```python
from build123d import *

# Parameters (mm, degrees)
SKETCH_1_W          = 450
SKETCH_1_H          = 400
EXTRUDE_1_DEPTH     = 6
SKETCH_3_R          = 3.75
SKETCH_3_R_2        = 4.25
CUT_EXTRUDE_2_DEPTH = 50
CUT_EXTRUDE_3_DEPTH = 50
SKETCH_5_W          = 45
SKETCH_5_H          = 45
CUT_EXTRUDE_4_DEPTH = 56
FILLET_1_R          = 5
SKETCH_6_R          = 4.25
CUT_EXTRUDE_5_DEPTH = 90


with BuildPart() as part:
    # 草图1 → 凸台-拉伸1 (new body)
    with BuildSketch(Plane.XY):
        Rectangle(SKETCH_1_W, SKETCH_1_H)
    extrude(amount=EXTRUDE_1_DEPTH)

    # 草图3 → 切除-拉伸2 (cut)
    with BuildSketch(Plane.XY.offset(6)):
        with Locations((205, -180)):
            Circle(SKETCH_3_R)
        with Locations((205, -120)):
            Circle(SKETCH_3_R_2)
        with Locations((145, -180)):
            Circle(SKETCH_3_R_2)
        with Locations((145, 180)):
            Circle(SKETCH_3_R_2)
        with Locations((205, 120)):
            Circle(SKETCH_3_R_2)
        with Locations((205, 180)):
            Circle(SKETCH_3_R)
        with Locations((-205, 180)):
            Circle(SKETCH_3_R)
        with Locations((-205, 120)):
            Circle(SKETCH_3_R_2)
        with Locations((-145, 180)):
            Circle(SKETCH_3_R_2)
        with Locations((-145, -180)):
            Circle(SKETCH_3_R_2)
        with Locations((-205, -120)):
            Circle(SKETCH_3_R_2)
        with Locations((-205, -180)):
            Circle(SKETCH_3_R)
    extrude(amount=-CUT_EXTRUDE_2_DEPTH, mode=Mode.SUBTRACT)

    # 草图4 → 切除-拉伸3 (cut)
    with BuildSketch(Plane.XY.offset(6)):
        with BuildLine():
            Line((100, -12.5), (-100, -12.5))
            ThreePointArc((-100, -12.5), (-112.5, 0), (-100, 12.5))
            Line((-100, 12.5), (100, 12.5))
            ThreePointArc((100, 12.5), (112.5, 0), (100, -12.5))
        make_face()
        with BuildLine():
            Line((100, 47.5), (-100, 47.5))
            ThreePointArc((-100, 47.5), (-112.5, 60), (-100, 72.5))
            Line((-100, 72.5), (100, 72.5))
            ThreePointArc((100, 72.5), (112.5, 60), (100, 47.5))
        make_face()
        with BuildLine():
            Line((100, -47.5), (-100, -47.5))
            ThreePointArc((-100, -47.5), (-112.5, -60), (-100, -72.5))
            Line((-100, -72.5), (100, -72.5))
            ThreePointArc((100, -72.5), (112.5, -60), (100, -47.5))
        make_face()
        with BuildLine():
            Line((100, 127.5), (-100, 127.5))
            ThreePointArc((-100, 127.5), (-112.5, 140), (-100, 152.5))
            Line((-100, 152.5), (100, 152.5))
            ThreePointArc((100, 152.5), (112.5, 140), (100, 127.5))
        make_face()
        with BuildLine():
            Line((100, -127.5), (-100, -127.5))
            ThreePointArc((-100, -127.5), (-112.5, -140), (-100, -152.5))
            Line((-100, -152.5), (100, -152.5))
            ThreePointArc((100, -152.5), (112.5, -140), (100, -127.5))
        make_face()
    extrude(amount=-CUT_EXTRUDE_3_DEPTH, mode=Mode.SUBTRACT)

    # 草图5 → 切除-拉伸4 (cut)
    with BuildSketch(Plane.XY.offset(6)):
        with Locations((202.5, -177.5)):
            Rectangle(SKETCH_5_W, SKETCH_5_H)
        with Locations((-202.5, -177.5)):
            Rectangle(SKETCH_5_W, SKETCH_5_H)
        with Locations((-202.5, 177.5)):
            Rectangle(SKETCH_5_W, SKETCH_5_H)
        with Locations((202.5, 177.5)):
            Rectangle(SKETCH_5_W, SKETCH_5_H)
    extrude(amount=-CUT_EXTRUDE_4_DEPTH, mode=Mode.SUBTRACT)

    # 圆角1
    fillet_1_edges = [part.edges().sort_by_distance(p)[0] for p in [
        (180, 200, 3),
        (225, 155, 3),
        (180, 155, 3),
        (-225, 155, 3),
        (-180, 200, 3),
        (-180, 155, 3),
        (-180, -200, 3),
        (-225, -155, 3),
        (-180, -155, 3),
        (225, -155, 3),
        (180, -200, 3),
        (180, -155, 3),
    ]]
    fillet(fillet_1_edges, radius=FILLET_1_R)

    # 草图6 → 切除-拉伸5 (cut)
    with BuildSketch(Plane(origin=(0, 0, 0), x_dir=(-1, 0, 0), z_dir=(0, 0, -1))):
        with Locations((15, -180)):
            Circle(SKETCH_6_R)
        with Locations((45, -180)):
            Circle(SKETCH_6_R)
        with Locations((75, -180)):
            Circle(SKETCH_6_R)
        with Locations((105, -180)):
            Circle(SKETCH_6_R)
        with Locations((-105, -180)):
            Circle(SKETCH_6_R)
        with Locations((-75, -180)):
            Circle(SKETCH_6_R)
        with Locations((-45, -180)):
            Circle(SKETCH_6_R)
        with Locations((-15, -180)):
            Circle(SKETCH_6_R)
        with Locations((-15, 180)):
            Circle(SKETCH_6_R)
        with Locations((-45, 180)):
            Circle(SKETCH_6_R)
        with Locations((-75, 180)):
            Circle(SKETCH_6_R)
        with Locations((-105, 180)):
            Circle(SKETCH_6_R)
        with Locations((105, 180)):
            Circle(SKETCH_6_R)
        with Locations((75, 180)):
            Circle(SKETCH_6_R)
        with Locations((45, 180)):
            Circle(SKETCH_6_R)
        with Locations((15, 180)):
            Circle(SKETCH_6_R)
        with Locations((-205, -12.5)):
            Circle(SKETCH_6_R)
        with Locations((-205, -37.5)):
            Circle(SKETCH_6_R)
        with Locations((-205, -62.5)):
            Circle(SKETCH_6_R)
        with Locations((-205, -87.5)):
            Circle(SKETCH_6_R)
        with Locations((-205, 87.5)):
            Circle(SKETCH_6_R)
        with Locations((-205, 62.5)):
            Circle(SKETCH_6_R)
        with Locations((-205, 37.5)):
            Circle(SKETCH_6_R)
        with Locations((-205, 12.5)):
            Circle(SKETCH_6_R)
        with Locations((205, 12.5)):
            Circle(SKETCH_6_R)
        with Locations((205, 37.5)):
            Circle(SKETCH_6_R)
        with Locations((205, 62.5)):
            Circle(SKETCH_6_R)
        with Locations((205, 87.5)):
            Circle(SKETCH_6_R)
        with Locations((205, -87.5)):
            Circle(SKETCH_6_R)
        with Locations((205, -62.5)):
            Circle(SKETCH_6_R)
        with Locations((205, -37.5)):
            Circle(SKETCH_6_R)
        with Locations((205, -12.5)):
            Circle(SKETCH_6_R)
    extrude(amount=-CUT_EXTRUDE_5_DEPTH, mode=Mode.SUBTRACT)


solid = part.part
```
Here's how the part is built. I have some questions about the finished solid (model axes, mm). A direction names the side the tool comes from. Coordinates: 2 decimals unless noted, no trailing zeros. Loops run counter-clockwise (first coordinate to the right, second up) from the corner with the lowest first, then second, coordinate; pieces in that order, holes last. Notation, with made-up numbers: (88.5, 35) - (127.5, 35) arc R21 cw to (127.5, 66) - close; hole circle Ø11 at (10, 64.25). An arc over 180 degrees is marked (long way). Return JSON: item names as keys, results as strings. Group by question number.
Item 1: If we section it at B-B on x = -193.5: Write out the boundary of the cut face in (y, z), and give its area (3 significant figures).
Item 2: On a 3-axis mill with a long thin cutter (end or side, diameter ignored), from which of +Z, -Z, +X, -X, +Y, -Y can I reach the whole of each face in a straight line? I mean faces 3 (the face through (-112.497, -0.275, 3.042)), 4 (the face through (-3, -42, 6)). Say none if no direction works.
Item 3: I need wall thicknesses on line 1 (Y direction, x = 84.5, z = 1.8); line 2 (X direction, y = 88, z = 1.1); line 3 (Y direction, x = 145, z = 1.35). Which ranges of each line are inside material? Lowest first, please. Write a range as from..to.
Item 4: We'd pull the mould along Y, two halves only. Please class faces 1 (the face through (-3, -42, 0)), 2 (the face through (112.497, 0.275, 3.042)): +Y half, -Y half, draft (parallel to the pull), parting line (faces both ways), or undercut.
Item 5: Will these pins go through, and if not, where does the flat tip stop? P1, Ø3, axis at y = 183, z = 4.5, coming from the +X side; P2, Ø4, axis at x = 73.5, y = 121, coming from the -Z side; P3, Ø7, axis at x = -205, y = 37.5, coming from the +Z side.
Item 6: If we section it at A-A on x = -85.5: Write out the boundary of the cut face in (y, z).
Calculated:
{
 "1": {"outline": "(-155, 0) - (155, 0) - (155, 6) - (-155, 6) - close", "area": "1,860 mm^2"},
 "2": {"face 3": "+Z, -Z", "face 4": "+Z, +X, -X, +Y, -Y"},
 "3": {"line 1": "y = -200..-152.5, -127.5..-72.5, -47.5..-12.5, 12.5..47.5, 72.5..127.5, 152.5..200", "line 2": "x = -225..-209.22, -200.78..200.78, 209.22..225", "line 3": "y = -200..-184.25, -175.75..175.75, 184.25..200"},
 "4": {"face 1": "draft", "face 2": "undercut"},
 "5": {"P1": "stops at x = 180", "P2": "stops at z = 0", "P3": "passes through"},
 "6": {"outline": "(-200, 0) - (-152.5, 0) - (-152.5, 6) - (-200, 6) - close; (-127.5, 0) - (-72.5, 0) - (-72.5, 6) - (-127.5, 6) - close; (-47.5, 0) - (-12.5, 0) - (-12.5, 6) - (-47.5, 6) - close; (12.5, 0) - (47.5, 0) - (47.5, 6) - (12.5, 6) - close; (72.5, 0) - (127.5, 0) - (127.5, 6) - (72.5, 6) - close; (152.5, 0) - (200, 0) - (200, 6) - (152.5, 6) - close"}
}
